```python
from build123d import *

# Parameters (mm, degrees)
SKETCH1_W                   = 1219.2
SKETCH1_H                   = 1974.85
BOSS_EXTRUDE1_DEPTH         = 6.35
SKETCH2_W                   = 533.4
SKETCH2_H                   = 457.2
SKETCH2_W_2                 = 355.6
SKETCH2_H_2                 = 355.6
CUT_EXTRUDE1_DEPTH          = 7.35
FILLET1_R                   = 6.35
F_1_4_0_25_DIAMETER_HOLE1_D = 6.35


with BuildPart() as part:
    # Sketch1 → Boss-Extrude1 (new body)
    with BuildSketch(Plane(origin=(0, 0, 0), x_dir=(0, 0, -1), z_dir=(1, 0, 0))):
        with Locations((609.6, 987.425)):
            Rectangle(SKETCH1_W, SKETCH1_H)
    extrude(amount=BOSS_EXTRUDE1_DEPTH)

    # Sketch2 → Cut-Extrude1 (cut, through all)
    with BuildSketch(Plane(origin=(6.35, 0, 0), x_dir=(0, 0, -1), z_dir=(1, 0, 0))):
        with Locations((777.875, 228.6)):
            Rectangle(SKETCH2_W, SKETCH2_H)
        with Locations((777.875, 685.8)):
            Rectangle(SKETCH2_W_2, SKETCH2_H_2)
    extrude(amount=-CUT_EXTRUDE1_DEPTH, mode=Mode.SUBTRACT)

    # Fillet1
    fillet1_edges = [part.edges().sort_by_distance(p)[0] for p in [
        (3.175, 457.2, -1044.575),
        (3.175, 457.2, -511.175),
        (3.175, 863.6, -955.675),
        (3.175, 508, -955.675),
        (3.175, 508, -600.075),
        (3.175, 863.6, -600.075),
    ]]
    fillet(fillet1_edges, radius=FILLET1_R)

    # 1/4 (0.25) Diameter Hole1 (through all)
    with Locations(Plane(origin=(6.35, 0, 0), x_dir=(0, 0, -1), z_dir=(1, 0, 0))):
        with Locations((1095.375, 57.15), (1095.375, 431.8), (1095.375, 876.3), (968.375, 844.55), (587.375, 844.55), (587.375, 527.05), (968.375, 527.05), (1016, 508), (1038.225, 876.3), (539.75, 508), (460.375, 431.8), (460.375, 57.15), (180.975, 876.3), (203.2, 508), (203.2, 450.85), (123.825, 876.3), (180.975, 57.15), (123.825, 57.15)):
            Hole(F_1_4_0_25_DIAMETER_HOLE1_D / 2)


solid = part.part
```
Model file for the job. Use its own axes, mm. Give positions to 0.01 mm unless a question says otherwise; leave off trailing zeros. Loops run counter-clockwise (first coordinate to the right, second up) from the corner with the lowest first, then second, coordinate; pieces in that order, holes last. Notation, with made-up numbers: M 42,31 L 47,31 A32 cw 47,62 Z; hole C 71.25,89.25 d7. An arc over 180 degrees is marked long. Use one line per item in the form item = value.
Item 1: Slice it at A-A on y = 231.5. List the corners of the cut face in (x, z) (3 decimals).
Filled in:
outline = M 0,-1219.2 L 6.35,-1219.2 L 6.35,-1044.575 L 0,-1044.575 Z; M 0,-511.175 L 6.35,-511.175 L 6.35,0 L 0,0 Z
Item 2: Drill centre lines: L1, parallel to Y at x = 2.75, z = -203; L2, parallel to Z at x = 4.75, y = 450.85 (3 decimals); L3, parallel to Z at x = 4.75, y = 527.05 (3 decimals). Where is each one in solid material? Low to high.
Filled in:
L1 = 0 to 447.68, 454.02 to 504.83, 511.17 to 1974.85
L2 = -1219.2 to -1044.575, -511.175 to -206.375, -200.025 to 0
L3 = -1219.2 to -971.55, -965.2 to -955.675, -600.075 to -590.55, -584.2 to 0
Item 3: Flat gauge pins, fed straight in: pin 1 Ø5 at (y, z) = (876.3, -1095.375) entering from -X; pin 2 Ø1.9 at (x, z) = (3, -845) entering from -Y. Where does each tip first touch, or does it go through?
Filled in:
pin_1 = through
pin_2 = 457.2
Item 4: Slice it at B-B on z = -764. List the corners of the cut face in (x, y).
Filled in:
outline = M 0,457.2 L 6.35,457.2 L 6.35,508 L 0,508 Z; M 0,863.6 L 6.35,863.6 L 6.35,1974.85 L 0,1974.85 Z
Item 5: Slice it at C-C on x = 4. Give the number of separate pieces and of enclosed holes in the cut face, and give its area (3 significant figures).
Filled in:
separate_pieces = 1
enclosed_holes = 19
area = 2,040,000 mm^2
